from build123d import *

# Parameters (mm, degrees)
F1_DEPTH = 300
F2_R     = 1
F3_R     = 2.38125


with BuildPart() as f1:
    # F0 (on Right) → F1 (new body, symmetric)
    with BuildSketch(Plane.YZ):
        Polygon((0, 25.4), (0, 0), (25.4, 0), (25.4, 4.7625), (4.7625, 4.7625), (4.7625, 25.4), align=None)
    extrude(amount=F1_DEPTH, both=True)

    # F2
    f2_edges = [f1.edges().sort_by_distance(p)[0] for p in [
        (0, 0, 25.4),
        (0, 4.7625, 25.4),
        (0, 0, 0),
        (0, 25.4, 4.7625),
        (0, 25.4, 0),
    ]]
    fillet(f2_edges, radius=F2_R)

    # F3
    f3_edges = [f1.edges().sort_by_distance(p)[0] for p in [
        (0, 4.7625, 4.7625),
    ]]
    fillet(f3_edges, radius=F3_R)


solid = f1.part
Work out the finished part from the listing and answer in its coordinate system (mm). A direction names the side the tool comes from. Coordinates: 2 decimals unless noted, no trailing zeros. Order: outer loops, then holes, each group sorted by start corner. A loop starts at its lowest first (then second) coordinate and runs counter-clockwise, first axis right, second up. Notation, with made-up numbers: (48, 79) - (89, 79) arc R32 ccw to (89, 118) - close; hole circle Ø6 at (52.25, 34.5). An arc over 180 degrees is marked (long way). Put each result on its own line as item: value. Start each with the question number.
1) Find section B-B (z = 11). Give the vertices of the cut face in (x, y).
2) Flat-ended cylindrical pins translate along their axes: pin 1 (3 mm diameter, centred on x = -99.5, z = 14.5, fed in from +Y); pin 2 (5 mm diameter, centred on x = 128, y = 15, fed in from +Z); pin 3 (10 mm diameter, centred on y = 5.5, z = 6.5, fed in from -X). Find the tip coordinate at first contact, or state that the pin passes through.
3) For faces 1 (the flat face through (-300, 4, 7)), 2 (the flat face through (4, 16, 4.762)), determine the directions among +Z, -Z, +X, -X, +Y, -Y from which every point of the face is accessible in a straight line to the end or side of a thin tool.
4) Find the intervals of material crossed by line 1 (Y direction, x = 20, z = 22.5), in increasing order. Write a range as from..to.
5) Find section A-A (x = -75). Give the vertices of the cut face in (y, z), plus the area to 3 significant figures.
Results list:
1. outline: (-300, 0) - (300, 0) - (300, 4.76) - (-300, 4.76) - close
2. pin 1: stops at y = 4.76
2. pin 2: stops at z = 4.76
2. pin 3: stops at x = -300
3. face 1: +Z, -Z, -X, +Y, -Y
3. face 2: +Z, +X, -X, +Y
4. line 1: y = 0..4.76
5. outline: (0, 1) arc R1 ccw to (1, 0) - (24.4, 0) arc R1 ccw to (25.4, 1) - (25.4, 3.76) arc R1 ccw to (24.4, 4.76) - (7.14, 4.76) arc R2.38 cw to (4.76, 7.14) - (4.76, 24.4) arc R1 ccw to (3.76, 25.4) - (1, 25.4) arc R1 ccw to (0, 24.4) - close
5. area: 219 mm^2
